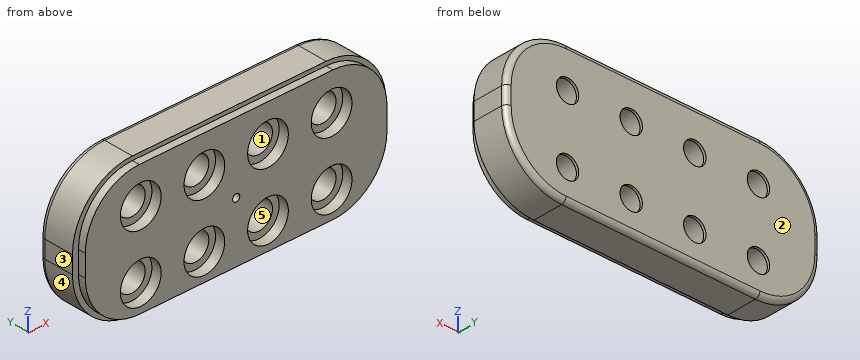
```python
from build123d import *

# Parameters (mm, degrees)
SKETCH1_W           = 16.0274
SKETCH1_H           = 7.0104
BOSS_EXTRUDE1_DEPTH = 1.778
SKETCH3_W           = 15.41526
SKETCH3_H           = 6.604
BOSS_EXTRUDE2_DEPTH = 0.381
FILLET2_R           = 2.7559
FILLET3_R           = 3.0607
SKETCH4_R           = 0.5715
CUT_EXTRUDE1_DEPTH  = 3.159
SKETCH5_R           = 0.6985
CUT_EXTRUDE2_DEPTH  = 2.032
SKETCH6_R           = 1.0414
CUT_EXTRUDE3_DEPTH  = 0.508
SKETCH7_R           = 0.18415
CUT_EXTRUDE4_DEPTH  = 0.508
FILLET4_R           = 0.254


with BuildPart() as part:
    # Sketch1 → Boss-Extrude1 (new body)
    with BuildSketch(Plane(origin=(0, 0, 0), x_dir=(1, 0, 0), z_dir=(0, 1, 0))):
        Rectangle(SKETCH1_W, SKETCH1_H)
    extrude(amount=BOSS_EXTRUDE1_DEPTH)

    # Sketch3 → Boss-Extrude2 (add)
    with BuildSketch(Plane.XZ):
        Rectangle(SKETCH3_W, SKETCH3_H)
    extrude(amount=BOSS_EXTRUDE2_DEPTH)

    # Fillet2
    fillet2_edges = [part.edges().sort_by_distance(p)[0] for p in [
        (-7.70763, -0.1905, 3.302),
        (-7.70763, -0.1905, -3.302),
        (7.70763, -0.1905, -3.302),
        (7.70763, -0.1905, 3.302),
    ]]
    fillet(fillet2_edges, radius=FILLET2_R)

    # Fillet3
    fillet3_edges = [part.edges().sort_by_distance(p)[0] for p in [
        (-8.0137, 0.889, -3.5052),
        (8.0137, 0.889, -3.5052),
        (8.0137, 0.889, 3.5052),
        (-8.0137, 0.889, 3.5052),
    ]]
    fillet(fillet3_edges, radius=FILLET3_R)

    # Sketch4 → Cut-Extrude1 (cut, through all)
    with BuildSketch(Plane(origin=(0, 1.778, 0), x_dir=(1, 0, 0), z_dir=(0, 1, 0))):
        with Locations((-4.8768, 1.9431)):
            Circle(SKETCH4_R)
        with Locations((-1.6256, 1.9431)):
            Circle(SKETCH4_R)
        with Locations((-4.8768, -1.4351)):
            Circle(SKETCH4_R)
        with Locations((-1.6256, -1.4351)):
            Circle(SKETCH4_R)
        with Locations((1.6256, -1.4351)):
            Circle(SKETCH4_R)
        with Locations((4.8768, -1.4351)):
            Circle(SKETCH4_R)
        with Locations((1.6256, 1.9431)):
            Circle(SKETCH4_R)
        with Locations((4.8768, 1.9431)):
            Circle(SKETCH4_R)
    extrude(amount=-CUT_EXTRUDE1_DEPTH, mode=Mode.SUBTRACT)

    # Sketch5 → Cut-Extrude2 (cut)
    with BuildSketch(Plane(origin=(0, -0.381, 0), x_dir=(1, 0, 0), z_dir=(0, 1, 0))):
        with Locations((-4.8768, -1.4351)):
            Circle(SKETCH5_R)
        with Locations((-4.8768, 1.9431)):
            Circle(SKETCH5_R)
        with Locations((-1.6256, 1.9431)):
            Circle(SKETCH5_R)
        with Locations((-1.6256, -1.4351)):
            Circle(SKETCH5_R)
        with Locations((1.6256, 1.9431)):
            Circle(SKETCH5_R)
        with Locations((1.6256, -1.4351)):
            Circle(SKETCH5_R)
        with Locations((4.8768, 1.9431)):
            Circle(SKETCH5_R)
        with Locations((4.8768, -1.4351)):
            Circle(SKETCH5_R)
    extrude(amount=CUT_EXTRUDE2_DEPTH, mode=Mode.SUBTRACT)

    # Sketch6 → Cut-Extrude3 (cut)
    with BuildSketch(Plane(origin=(0, -0.381, 0), x_dir=(1, 0, 0), z_dir=(0, 1, 0))):
        with Locations((-4.8768, 1.9431)):
            Circle(SKETCH6_R)
        with Locations((-4.8768, -1.4351)):
            Circle(SKETCH6_R)
        with Locations((-1.6256, -1.4351)):
            Circle(SKETCH6_R)
        with Locations((-1.6256, 1.9431)):
            Circle(SKETCH6_R)
        with Locations((1.6256, 1.9431)):
            Circle(SKETCH6_R)
        with Locations((1.6256, -1.4351)):
            Circle(SKETCH6_R)
        with Locations((4.8768, -1.4351)):
            Circle(SKETCH6_R)
        with Locations((4.8768, 1.9431)):
            Circle(SKETCH6_R)
    extrude(amount=CUT_EXTRUDE3_DEPTH, mode=Mode.SUBTRACT)

    # Sketch7 → Cut-Extrude4 (cut)
    with BuildSketch(Plane.XZ.offset(0.381)):
        with Locations((0, -0.254)):
            Circle(SKETCH7_R)
    extrude(amount=-CUT_EXTRUDE4_DEPTH, mode=Mode.SUBTRACT)

    # Fillet4
    fillet4_edges = [part.edges().sort_by_distance(p)[0] for p in [
        (0, 1.778, 3.5052),
        (-8.0137, 1.778, 0),
        (8.0137, 1.778, 0),
        (0, 1.778, -3.5052),
        (7.117241725, 1.778, -2.608741725),
        (7.117241725, 1.778, 2.608741725),
        (-7.117241725, 1.778, -2.608741725),
        (-7.117241725, 1.778, 2.608741725),
    ]]
    fillet(fillet4_edges, radius=FILLET4_R)


solid = part.part
```
Read the model definition and answer for the solid it produces. Units are mm, in the model's axes. Face numbers are marked on the shaded views. A direction names the side the tool comes from. Round coordinates to 2 decimals unless told otherwise and drop trailing zeros. Write each loop counter-clockwise with the first axis right and the second up, starting at its lowest first coordinate (ties: lowest second). Pieces come first, ordered by that corner, then holes. Notation, with made-up numbers: (5.5, 10) -> (55.5, 10) arc R12 cw to (55.5, 33) -> close; hole circle Ø8 at (76, 24). An arc over 180 degrees is marked (long way). Answer in a Markdown table with one row per item. Add a question column.
1) Given P1, Ø1, axis at x = 5, z = -2, coming from the -Y side; P2, Ø0.7, axis at x = 1.5, z = 1.5, coming from the -Y side; P3, Ø1.7, axis at x = 5, z = 1.5, coming from the -Y side, each flat-ended and moving along its own axis, determine where each tip first touches the part or whether it passes through.
2) Which of the six approach directions +Z, -Z, +X, -X, +Y, -Y give full straight-line access (tool end or side, diameter ignored) to the marked faces 4 and 5?
3) Find section A-A, the plane x = 0. Determine the outline of the cut face in (y, z).
4) Consider line 1 (X direction, y = 1.4, z = 1.75); line 2 (X direction, y = 1.3, z = 1.5); line 3 (Z direction, x = -2, y = 0.9). Determine where each line is inside the solid, lowest interval first.
5) Find section B-B, the plane y = 0.4. State how many separate pieces and enclosed holes the cut face has, and give its area (3 significant figures).
6) Determine the mould class of the marked faces 1, 2 and 3 for opening direction X: pulls with the +X half, pulls with the -X half, needs draft (parallel to the pull), parting line crosses it, or undercut.
Findings below:
| question | item | result |
|---|---|---|
| 1 | P1 | y = 1.65 |
| 1 | P2 | through |
| 1 | P3 | y = 0.13 |
| 2 | face 4 | -Z, -X, +Y, -Y |
| 2 | face 5 | -Y |
| 3 | outline | (-0.38, -3.3) -> (0, -3.3) -> (0, -3.51) -> (1.52, -3.51) arc R0.25 ccw to (1.78, -3.25) -> (1.78, 3.25) arc R0.25 ccw to (1.52, 3.51) -> (0, 3.51) -> (0, 3.3) -> (-0.38, 3.3) -> (-0.38, -0.07) -> (0.13, -0.07) -> (0.13, -0.44) -> (-0.38, -0.44) -> close |
| 4 | line 1 | -7.72 to -5.5, -4.25 to -2.25, -1 to 1, 2.25 to 4.25, 5.5 to 7.72 |
| 4 | line 2 | -7.83 to -5.57, -4.18 to -2.32, -0.93 to 0.93, 2.32 to 4.18, 5.57 to 7.83 |
| 4 | line 3 | -3.51 to -2.53, -1.35 to 0.85, 2.02 to 3.51 |
| 5 | separate pieces | 1 |
| 5 | enclosed holes | 8 |
| 5 | area | 92.1 mm² |
| 6 | face 1 | undercut |
| 6 | face 2 | needs draft |
| 6 | face 3 | pulls with the -X half |
